from build123d import *

# Parameters (mm, degrees)
F1_DEPTH = 25.4


with BuildPart() as f1:
    # F0 (on Front) → F1 (new body)
    with BuildSketch(Plane.XZ):
        with BuildLine():
            ThreePointArc((46.1673500078, -15.2324506451), (47.999444804, -7.7139521587), (48.6153448964, 0))
            ThreePointArc((48.6153448964, 0), (46.4980117159, 14.1910769804), (40.3304436459, 27.1460323938))
            add(Edge.make_bspline(
                [(40.3304436459, 27.1460323938), (32.3786976376, 23.0993060038), (24.4227156617, 19.0482632148), (16.5014874139, 16.4513327342)],
                knots=[0, 0, 0, 0, 0.2953409121, 0.2953409121, 0.2953409121, 0.2953409121], degree=3))
            add(Edge.make_bspline(
                [(16.5014873898, 16.4513327474), (15.5953694896, 11.2931775522), (15.5320066906, 3.0058951007), (18.67748395, -6.2871122776), (19.9799499764, -9.4342211392)],
                knots=[0.2963486373, 0.2963486373, 0.2963486373, 0.2963486373, 0.4715656378, 0.5637333, 0.5637333, 0.5637333, 0.5637333], degree=3))
            add(Edge.make_bspline(
                [(46.1673500078, -15.2324506451), (37.3947505843, -12.9712227578), (28.6158550244, -10.7067465721), (19.9799499764, -9.4342211392)],
                knots=[0, 0, 0, 0, 0.282903213, 0.282903213, 0.282903213, 0.282903213], degree=3))
        make_face()
        with BuildLine():
            add(Edge.make_bspline(
                [(40.3304436459, 27.1460323938), (32.3786976376, 23.0993060038), (24.4227156617, 19.0482632148), (16.5014874139, 16.4513327342)],
                knots=[0, 0, 0, 0, 0.2953409121, 0.2953409121, 0.2953409121, 0.2953409121], degree=3))
            ThreePointArc((40.3304436459, 27.1460323938), (33.903902399, 34.84217504), (26.0352353751, 41.056281838))
            add(Edge.make_bspline(
                [(26.0352353751, 41.056281838), (22.0398072792, 33.1200566973), (18.0340259226, 25.1754420421), (16.5014873898, 16.4513327474)],
                knots=[0, 0, 0, 0, 0.2963486373, 0.2963486373, 0.2963486373, 0.2963486373], degree=3))
        make_face()
        with BuildLine():
            ThreePointArc((36.2646535731, -32.3778730095), (42.0981018646, -24.3146371306), (46.1673500078, -15.2324506451))
            add(Edge.make_bspline(
                [(46.1673500078, -15.2324506451), (37.3947505843, -12.9712227578), (28.6158550244, -10.7067465721), (19.9799499764, -9.4342211392)],
                knots=[0, 0, 0, 0, 0.282903213, 0.282903213, 0.282903213, 0.282903213], degree=3))
            add(Edge.make_bspline(
                [(19.9799499764, -9.4342211392), (25.0191791568, -21.6103566301), (33.3249337281, -32.9452793274), (35.454034531, -33.2635415263)],
                knots=[0.5637333, 0.5637333, 0.5637333, 0.5637333, 0.9203291446, 0.9203291446, 0.9203291446, 0.9203291446], degree=3))
            ThreePointArc((35.454034531, -33.2635415263), (35.8620782725, -32.823209797), (36.2646535731, -32.3778730095))
        make_face()
        with BuildLine():
            add(Edge.make_bspline(
                [(26.0352353751, 41.056281838), (22.0398072792, 33.1200566973), (18.0340259226, 25.1754420421), (16.5014873898, 16.4513327474)],
                knots=[0, 0, 0, 0, 0.2963486373, 0.2963486373, 0.2963486373, 0.2963486373], degree=3))
            ThreePointArc((26.0352353751, 41.056281838), (-1.9947078477, 48.5744058121), (-29.3138505417, 38.7833717695))
            add(Edge.make_bspline(
                [(-29.3138505417, 38.7833717695), (-27.000307279, 32.4407823134), (-24.6802191732, 26.0937743503), (-22.973223534, 19.7963497545)],
                knots=[0, 0, 0, 0, 0.2452233004, 0.2452233004, 0.2452233004, 0.2452233004], degree=3))
            add(Edge.make_bspline(
                [(16.5014874139, 16.4513327342), (10.9797013124, 14.6410459723), (-2.2734109483, 11.9838999083), (-15.3520884673, 16.285685391), (-22.973223534, 19.7963497545)],
                knots=[0.2953409121, 0.2953409121, 0.2953409121, 0.2953409121, 0.5012192547, 0.7909956335, 0.7909956335, 0.7909956335, 0.7909956335], degree=3))
        make_face()
        with BuildLine():
            add(Edge.make_bspline(
                [(16.5014873898, 16.4513327474), (15.5953694896, 11.2931775522), (15.5320066906, 3.0058951007), (18.67748395, -6.2871122776), (19.9799499764, -9.4342211392)],
                knots=[0.2963486373, 0.2963486373, 0.2963486373, 0.2963486373, 0.4715656378, 0.5637333, 0.5637333, 0.5637333, 0.5637333], degree=3))
            add(Edge.make_bspline(
                [(16.5014874139, 16.4513327342), (10.9797013124, 14.6410459723), (-2.2734109483, 11.9838999083), (-15.3520884673, 16.285685391), (-22.973223534, 19.7963497545)],
                knots=[0.2953409121, 0.2953409121, 0.2953409121, 0.2953409121, 0.5012192547, 0.7909956335, 0.7909956335, 0.7909956335, 0.7909956335], degree=3))
            add(Edge.make_bspline(
                [(-22.973223534, 19.7963497545), (-21.1636232806, 13.1203976417), (-19.1493739324, 1.2205893586), (-21.7464907751, -10.2913075482), (-23.4240943414, -15.3533007473)],
                knots=[0.2452233004, 0.2452233004, 0.2452233004, 0.2452233004, 0.5051865577, 0.7125051709, 0.7125051709, 0.7125051709, 0.7125051709], degree=3))
            add(Edge.make_bspline(
                [(19.9799499764, -9.4342211392), (13.2080472289, -8.4363618033), (-1.6767781675, -7.5725154611), (-15.7685768428, -12.1133609217), (-23.4240943551, -15.3533007369)],
                knots=[0.282903213, 0.282903213, 0.282903213, 0.282903213, 0.5047436611, 0.776928854, 0.776928854, 0.776928854, 0.776928854], degree=3))
        make_face()
        with BuildLine():
            add(Edge.make_bspline(
                [(19.9799499764, -9.4342211392), (25.0191791568, -21.6103566301), (33.3249337281, -32.9452793274), (35.454034531, -33.2635415263)],
                knots=[0.5637333, 0.5637333, 0.5637333, 0.5637333, 0.9203291446, 0.9203291446, 0.9203291446, 0.9203291446], degree=3))
            add(Edge.make_bspline(
                [(19.9799499764, -9.4342211392), (13.2080472289, -8.4363618033), (-1.6767781675, -7.5725154611), (-15.7685768428, -12.1133609217), (-23.4240943551, -15.3533007369)],
                knots=[0.282903213, 0.282903213, 0.282903213, 0.282903213, 0.5047436611, 0.776928854, 0.776928854, 0.776928854, 0.776928854], degree=3))
            add(Edge.make_bspline(
                [(-23.4240943414, -15.3533007473), (-25.7504766345, -22.3729158592), (-29.0871025112, -29.3050684982), (-32.4143035176, -36.2320947071)],
                knots=[0.7125051709, 0.7125051709, 0.7125051709, 0.7125051709, 1, 1, 1, 1], degree=3))
            ThreePointArc((-32.4143035176, -36.2320947071), (2.1243983043, -48.5689066301), (35.454034531, -33.2635415263))
        make_face()
        with BuildLine():
            add(Edge.make_bspline(
                [(-22.973223534, 19.7963497545), (-21.1636232806, 13.1203976417), (-19.1493739324, 1.2205893586), (-21.7464907751, -10.2913075482), (-23.4240943414, -15.3533007473)],
                knots=[0.2452233004, 0.2452233004, 0.2452233004, 0.2452233004, 0.5051865577, 0.7125051709, 0.7125051709, 0.7125051709, 0.7125051709], degree=3))
            add(Edge.make_bspline(
                [(-22.973223534, 19.7963497545), (-28.4700501333, 22.3284546294), (-33.9538200156, 25.3785378793), (-39.4374864795, 28.4277403178)],
                knots=[0.7909956335, 0.7909956335, 0.7909956335, 0.7909956335, 1, 1, 1, 1], degree=3))
            ThreePointArc((-39.4374864795, 28.4277403178), (-48.5534662677, 2.4520752004), (-42.1008703821, -24.3098431189))
            add(Edge.make_bspline(
                [(-23.4240943551, -15.3533007369), (-29.6982235487, -18.0086144957), (-35.899537129, -21.1597200741), (-42.1008703821, -24.3098431189)],
                knots=[0.776928854, 0.776928854, 0.776928854, 0.776928854, 1, 1, 1, 1], degree=3))
        make_face()
        with BuildLine():
            add(Edge.make_bspline(
                [(-23.4240943414, -15.3533007473), (-25.7504766345, -22.3729158592), (-29.0871025112, -29.3050684982), (-32.4143035176, -36.2320947071)],
                knots=[0.7125051709, 0.7125051709, 0.7125051709, 0.7125051709, 1, 1, 1, 1], degree=3))
            add(Edge.make_bspline(
                [(-23.4240943551, -15.3533007369), (-29.6982235487, -18.0086144957), (-35.899537129, -21.1597200741), (-42.1008703821, -24.3098431189)],
                knots=[0.776928854, 0.776928854, 0.776928854, 0.776928854, 1, 1, 1, 1], degree=3))
            ThreePointArc((-42.1008703821, -24.3098431189), (-37.731456453, -30.6559774487), (-32.4143035176, -36.2320947071))
        make_face()
    extrude(amount=F1_DEPTH)


solid = f1.part
The model under review builds one solid part; all positions refer to its coordinate system, in mm. Round coordinates to 2 decimals unless told otherwise and drop trailing zeros. Write each loop counter-clockwise with the first axis right and the second up, starting at its lowest first coordinate (ties: lowest second). Pieces come first, ordered by that corner, then holes. Notation, with made-up numbers: (-25, -12) -> (24, -12) arc R20 cw to (24, 17) -> close; hole circle Ø1 at (-2.5, 3). An arc over 180 degrees is marked (long way). Answer as a JSON object with one key per item and string values.
1. Clearance check with flat-ended pins moving along their axes: pin 1 (12 mm diameter, centred on x = 13, y = -17.5, fed in from +Z); pin 2 (5 mm diameter, centred on x = 11, y = -6, fed in from -Z); pin 3 (4 mm diameter, centred on x = -14, y = -2.5, fed in from +Z). State where each tip first meets the part, or that it passes through.
Results found:
{"pin 1": "stops at z = 48.11", "pin 2": "stops at z = -47.87", "pin 3": "stops at z = 47.11"}
2. We need section A-A on z = -11. State the section outline as (x, y) points, and give its area (3 significant figures).
Results found:
{"outline": "(-47.35, -25.4) -> (47.35, -25.4) -> (47.35, 0) -> (-47.35, 0) -> close", "area": "2,410 mm^2"}
3. To check wall thickness, follow line 1 along Z through (x, y) = (-1, -15); line 2 along X through (y, z) = (-17.25, 21.5); line 3 along X through (y, z) = (-14, 25.5). State the ranges of each line that lie inside material, in increasing order.
Results found:
{"line 1": "z = -48.61 to 48.61", "line 2": "x = -43.6 to -26.52, -23.45 to 43.6", "line 3": "x = -41.39 to -34.14, -24.67 to 41.39"}
4. We need section B-B on x = 28.5. State the section outline as (y, z) points, and give its area (3 significant figures).
Results found:
{"outline": "(-25.4, -39.39) -> (0, -39.39) -> (0, 39.39) -> (-25.4, 39.39) -> close", "area": "2,000 mm^2"}
